```python
from build123d import *

# Parameters (mm, degrees)
F0_W     = 88.9
F0_H     = 88.9
F1_DEPTH = 304.8
F2_W     = 31.75
F2_H     = 114.3
F3_DEPTH = 127
F4_R     = 6.35
F5_DEPTH = 127


with BuildPart() as f1:
    # F0 (on Front) → F1 (new body)
    with BuildSketch(Plane.XZ):
        with Locations((1.7375517637, 8.7750459692)):
            Rectangle(F0_W, F0_H)
    extrude(amount=F1_DEPTH)

    # F2 (on Top) → F3 (cut, symmetric)
    with BuildSketch(Plane.XY):
        with Locations((-26.8374482363, -57.15)):
            Rectangle(F2_W, F2_H)
        with Locations((30.3125517637, -57.15)):
            Rectangle(F2_W, F2_H)
    extrude(amount=F3_DEPTH, both=True, mode=Mode.SUBTRACT)

    # F4 (on face) → F5 (cut, symmetric)
    with BuildSketch(Plane.YZ.offset(14.4375517637)):
        with Locations((-44.45, 8.7750459692)):
            Circle(F4_R)
    extrude(amount=F5_DEPTH, both=True, mode=Mode.SUBTRACT)


solid = f1.part
```
Geometry: final body of the model. Coordinates: model frame, mm. A direction names the side the tool comes from. Coordinates: 2 decimals unless noted, no trailing zeros. Order: outer loops, then holes, each group sorted by start corner. A loop starts at its lowest first (then second) coordinate and runs counter-clockwise, first axis right, second up. Notation, with made-up numbers: (23, -10.5) -> (55, -10.5) arc R24 ccw to (55, 6.5) -> close; hole circle Ø4 at (14.5, -36). An arc over 180 degrees is marked (long way). Use CSV: the item, a comma, the result in double quotes.
1) Line query: line 1 (Z direction, x = 0.75, y = -44.45); line 2 (Y direction, x = 28.5, z = -23.5); line 3 (X direction, y = -78.5, z = 43.5). Output: solid intervals per line, ascending.
Findings:
line 1,"z = -35.67 to 2.43, 15.13 to 53.23"
line 2,"y = -304.8 to -114.3"
line 3,"x = -10.96 to 14.44"
2) Section C-C on x = -26. Output: boundary loops of the cut face in (y, z).
Findings:
outline,"(-304.8, -35.67) -> (-114.3, -35.67) -> (-114.3, 53.23) -> (-304.8, 53.23) -> close"
3) Pin query (flat end, axial travel): pin 1 Ø20.5 at (y, z) = (-44.45, 8.78) entering from -X; pin 2 Ø16 at (x, z) = (28.5, 20) entering from +Y. Return the tip coordinate at first contact, or that it passes through.
Findings:
pin 1,"stops at x = -10.96"
pin 2,"stops at y = -114.3"
4) Section A-A on y = -44.45. Output: boundary loops of the cut face in (x, z).
Findings:
outline,"(-10.96, -35.67) -> (14.44, -35.67) -> (14.44, 2.43) -> (-10.96, 2.43) -> close; (-10.96, 15.13) -> (14.44, 15.13) -> (14.44, 53.23) -> (-10.96, 53.23) -> close"
5) Mould query, pull axis Y, two halves, no side actions, for faces 1 (the flat face through (30, -114.3, 9)), 2 (the flat face through (1, -304.8, 9)), 3 (the cylindrical face through (1.9, -38.4, 10.7)). Classes: +Y half, -Y half, draft (parallel to the pull), parting line (faces both ways), or undercut.
Findings:
face 1,"+Y half"
face 2,"-Y half"
face 3,"undercut"
6) Access query for faces 4 (the flat face through (14.438, -58, 9)), 5 (the flat face through (-10.962, -58, 8)), 6 (the flat face through (1, -184, -35.675)). Directions: +Z, -Z, +X, -X, +Y, -Y. A direction counts if a zero-diameter tool reaches every point of the face in a straight line with its end or side. Return the directions, or none.
Findings:
face 4,"+Z, -Z, +X, +Y"
face 5,"+Z, -Z, -X, +Y"
face 6,"-Z, +X, -X, +Y, -Y"
7) Section B-B on z = 29.5. Output: boundary loops of the cut face in (x, y).
Findings:
outline,"(-42.71, -304.8) -> (46.19, -304.8) -> (46.19, -114.3) -> (14.44, -114.3) -> (14.44, 0) -> (-10.96, 0) -> (-10.96, -114.3) -> (-42.71, -114.3) -> close"
